from build123d import *

# Parameters (mm, degrees)
F0_R     = 28.6512
F1_DEPTH = 83.058
F2_W     = 18.0594
F2_H     = 15.9512
F4_DEPTH = 60.706


# Not quite as in the source:
# - a feature of the source that left no trace in its solid (it failed there, or was rolled back) is left out


with BuildPart() as f1:
    # F0 (on Top) → F1 (new body, symmetric)
    with BuildSketch(Plane.XY):
        Circle(F0_R)
    extrude(amount=F1_DEPTH, both=True)

    # F2 (on Right) → F4 (cut)
    with BuildSketch(Plane.YZ):
        with Locations((9.0297, 7.9756)):
            Rectangle(F2_W, F2_H)
    extrude(amount=-F4_DEPTH, mode=Mode.SUBTRACT)


solid = f1.part
Can you work these out from the model? Positions are in its coordinate system, mm. A direction names the side the tool comes from. Coordinates: 2 decimals unless noted, no trailing zeros. Write each loop counter-clockwise with the first axis right and the second up, starting at its lowest first coordinate (ties: lowest second). Pieces come first, ordered by that corner, then holes. Notation, with made-up numbers: (-12.75, 0) -> (-1.75, 0) arc R18 cw to (-1.75, 13) -> close; hole circle Ø10 at (-22.75, -28). An arc over 180 degrees is marked (long way). Write each question's results on one line, items separated by ' | '. Start each with the question number.
Item 1: If we section it at D-D, the plane x = 12.5: Write out the boundary of the cut face in (y, z).
Item 2: If we section it at C-C, the plane z = -18: Write out the boundary of the cut face in (x, y), and give its area (3 significant figures).
Item 3: Please list where these lines run through material, in increasing order: probe 1 along Z at (x, y) = (-23, 3.5); probe 2 along Y at (x, z) = (1, 12.5).
Item 4: Thinking about a two-plate mould opening in Z: for faces 3 (the cylindrical face through (26.47, -10.97, 1.16)), 4 (the flat face through (-11, 18.059, 8)), 5 (the flat face through (0, 9, 8)), 6 (the flat face through (0, 0, 83.058)), which applies, released by +Z, released by -Z, zero draft, split by the parting line, or undercut?
Item 5: If we section it at A-A, the plane x = -10: Write out the boundary of the cut face in (y, z).
Item 6: I'm going to push flat-ended pins straight in: P1, Ø3, axis at y = -1, z = -10.5, coming from the +X side; P2, Ø17.5, axis at x = -10, z = 8.5, coming from the -Y side; P3, Ø5, axis at y = -19, z = -9.5, coming from the +X side; P4, Ø4, axis at x = -4, z = -54, coming from the +Y side. Where does each tip first touch, or does it pass through?
Item 7: If we section it at B-B, the plane y = 4: Write out the boundary of the cut face in (x, z).
Item 8: On a 3-axis mill with a long thin cutter (end or side, diameter ignored), from which of +Z, -Z, +X, -X, +Y, -Y can I reach the whole of each face in a straight line? I mean faces 1 (the flat face through (0, 0, -83.058)), 2 (the flat face through (-14, 9, 15.951)). Say none if no direction works.
Answer block:
1) outline: (-25.78, -83.06) -> (25.78, -83.06) -> (25.78, 83.06) -> (-25.78, 83.06) -> close
2) outline: circle Ø57.3 at (0, 0) | area: 2,580 mm²
3) probe 1: -83.06 to 0, 15.95 to 83.06 | probe 2: -28.63 to 28.63
4) face 3: zero draft | face 4: undercut | face 5: undercut | face 6: released by +Z
5) outline: (-26.85, -83.06) -> (26.85, -83.06) -> (26.85, 83.06) -> (-26.85, 83.06) -> close; hole (0, 0) -> (18.06, 0) -> (18.06, 15.95) -> (0, 15.95) -> close
6) P1: x = 28.65 | P2: y = -28.62 | P3: x = 23.42 | P4: y = 28.58
7) outline: (-28.37, -83.06) -> (28.37, -83.06) -> (28.37, 83.06) -> (-28.37, 83.06) -> (-28.37, 15.95) -> (0, 15.95) -> (0, 0) -> (-28.37, 0) -> close
8) face 1: -Z, +X, -X, +Y, -Y | face 2: -X
